Source: three-view drawing plus pictorial views. Frame: mm from the lowest corner of the part. A direction names the side the tool comes from. Give positions to 0.01 mm unless a question says otherwise; leave off trailing zeros. Order: outer loops, then holes, each group sorted by start corner. A loop starts at its lowest first (then second) coordinate and runs counter-clockwise, first axis right, second up. Notation, with made-up numbers: (-35, 66.25) - (-22, 66.25) arc R27 ccw to (-22, 99.25) - close; hole circle Ø4 at (-9, 26.5). An arc over 180 degrees is marked (long way). Use CSV: the item, a comma, the result in double quotes.
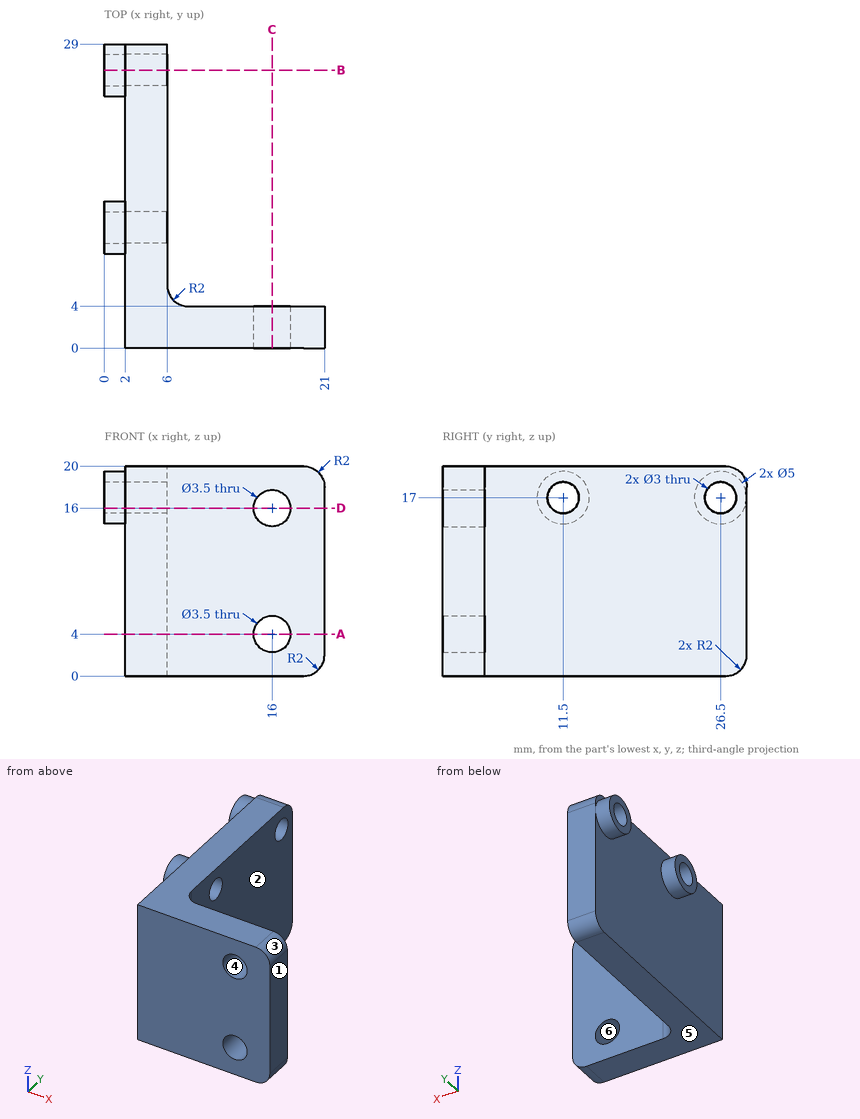
Item 1: Set-up query: the marked faces 1 and 2. Return all of +Z, -Z, +X, -X, +Y, -Y with unobstructed straight access to the full face (end or side cutting, diameter ignored); none if empty.
Filled in:
face 1,"+Z, -Z, +X, +Y, -Y"
face 2,"+Z, -Z, +X, +Y"
Item 2: Section B-B on y = 26.5. Return the cut outline in (x, z).
Filled in:
outline,"(0, 14.5) - (2, 14.5) - (2, 0) - (6, 0) - (6, 15.5) - (0, 15.5) - close; (0, 18.5) - (6, 18.5) - (6, 20) - (2, 20) - (2, 19.5) - (0, 19.5) - close"
Item 3: Material intervals for line 1 (Y direction, x = 0.55, z = 17); line 2 (Y direction, x = 3.75, z = 17); line 3 (Z direction, x = 3.95, y = 11.5), sorted ascending. Write a range as from..to.
Filled in:
line 1,"y = 9..10, 13..14, 24..25, 28..29"
line 2,"y = 0..10, 13..25, 28..29"
line 3,"z = 0..15.5, 18.5..20"
Item 4: Section D-D on z = 16. Return the cut outline in (x, y), then the cut area to 3 significant figures.
Filled in:
outline,"(0, 9.21) - (2, 9.21) - (2, 0) - (14.25, 0) - (14.25, 4) - (8, 4) arc R2 cw to (6, 6) - (6, 10.38) - (0, 10.38) - close; (0, 12.62) - (6, 12.62) - (6, 25.38) - (0, 25.38) - (0, 24.21) - (2, 24.21) - (2, 13.79) - (0, 13.79) - close; (0, 27.62) - (6, 27.62) - (6, 29) - (2, 29) - (2, 28.79) - (0, 28.79) - close; (17.75, 0) - (21, 0) - (21, 4) - (17.75, 4) - close"
area,"154 mm2"
Item 5: Section C-C on x = 16. Return the cut outline in (y, z), then the cut area to 3 significant figures.
Filled in:
outline,"(0, 0) - (4, 0) - (4, 2.25) - (0, 2.25) - close; (0, 5.75) - (4, 5.75) - (4, 14.25) - (0, 14.25) - close; (0, 17.75) - (4, 17.75) - (4, 20) - (0, 20) - close"
area,"52.0 mm2"
Item 6: Mould query, pull axis Z, two halves, no side actions, for the marked faces 3, 4, 5 and 6. Classes: released by +Z, released by -Z, zero draft, split by the parting line, or undercut.
Filled in:
face 3,"released by +Z"
face 4,"undercut"
face 5,"released by -Z"
face 6,"undercut"
Item 7: First-contact query: pin 1 (10 mm diameter, centred on y = 22, z = 5.5, fed in from +X); pin 2 (6.5 mm diameter, centred on x = 15.5, z = 10, fed in from +Y). Flat tips, straight axial feed; report the tip coordinate or a pass-through.
Filled in:
pin 1,"stops at x = 6"
pin 2,"stops at y = 4"
Item 8: Section A-A on z = 4. Return the cut outline in (x, y), then the cut area to 3 significant figures.
Filled in:
outline,"(2, 0) - (14.25, 0) - (14.25, 4) - (8, 4) arc R2 cw to (6, 6) - (6, 29) - (2, 29) - close; (17.75, 0) - (21, 0) - (21, 4) - (17.75, 4) - close"
area,"163 mm2"
